from build123d import *

# Parameters (mm, degrees)
REVOLVE1_ANGLE           = 175
REVOLVE1_OTHER_WAY_ANGLE = 175
BOSS_EXTRUDE1_DEPTH      = 1.75
SKETCH5_R                = 1
BOSS_EXTRUDE2_DEPTH      = 3
FILLET1_R                = 1
FILLET1_OF_MIRROR1_R     = 1


with BuildPart() as part:
    # Sketch2 → Revolve1 (revolve)
    with BuildSketch(Plane(origin=(0, 0, 0), x_dir=(0, 0, -1), z_dir=(1, 0, 0))):
        Polygon((1.75, -70), (1.75, -71.8), (1.5, -71.8), (0.5, -73), (-0.5, -73), (-1.5, -71.8), (-1.75, -71.8), (-1.75, -70), align=None)
    revolve(axis=Axis((0, 0, 0), (0, 0, -1)), revolution_arc=REVOLVE1_ANGLE)

    # Sketch2 → Revolve1 other way (revolve)
    with BuildSketch(Plane(origin=(0, 0, 0), x_dir=(0, 0, -1), z_dir=(1, 0, 0))):
        Polygon((1.75, -70), (1.75, -71.8), (1.5, -71.8), (0.5, -73), (-0.5, -73), (-1.5, -71.8), (-1.75, -71.8), (-1.75, -70), align=None)
    revolve(axis=Axis((0, 0, 0), (0, 0, 1)), revolution_arc=REVOLVE1_OTHER_WAY_ANGLE)

    # Sketch3 → Boss-Extrude1 (add, symmetric)
    with BuildSketch(Plane.XY):
        Polygon((-70, 0), (-20, 0), (-20, -3), (-51, -3), (-68.736443607, -13.240140491), (-69.736443607, -11.508089684), (-55, -3), (-70, -3), align=None)
    boss_extrude1 = extrude(amount=BOSS_EXTRUDE1_DEPTH, both=True)

    # Sketch5 → Boss-Extrude2 (add)
    with BuildSketch(Plane(origin=(-20, 0, 0), x_dir=(0, 0, -1), z_dir=(1, 0, 0))):
        with Locations((0, -1.5)):
            Circle(SKETCH5_R)
    boss_extrude2 = extrude(amount=BOSS_EXTRUDE2_DEPTH)

    # Fillet1
    fillet1_edges = [part.edges().sort_by_distance(p)[0] for p in [
        (-69.93568474, -3, 0),
        (-69.107123463, -11.144751529, 0),
        (-70, 0, 0),
        (-55, -3, 0),
        (-51, -3, 0),
    ]]
    fillet(fillet1_edges, radius=FILLET1_R)

    # Mirror1: Boss-Extrude1, Boss-Extrude2 across plane
    add(boss_extrude1.mirror(Plane(origin=(0, 0, 0), x_dir=(0, 0, 1), z_dir=(1, 0, 0))))
    add(boss_extrude2.mirror(Plane(origin=(0, 0, 0), x_dir=(0, 0, 1), z_dir=(1, 0, 0))))

    # Fillet1 of Mirror1
    fillet1_of_mirror1_edges = [part.edges().sort_by_distance(p)[0] for p in [
        (69.93568474, -3, 0),
        (69.107123463, -11.144751529, 0),
        (70, 0, 0),
        (55, -3, 0),
        (51, -3, 0),
    ]]
    fillet(fillet1_of_mirror1_edges, radius=FILLET1_OF_MIRROR1_R)


solid = part.part
Verification items for the finished model (mm, model axes). A direction names the side the tool comes from. Give positions to 0.01 mm unless a question says otherwise; leave off trailing zeros. Use CSV: the item, a comma, the result in double quotes.
1) Release check for a two-part mould opening along X. For faces 1 (the face through (58, -5, -1.75)), 2 (the face through (-45, 0, 0)), 3 (the face through (-3.077, -71.926, 1.34)) record: released by +X, released by -X, zero draft, split by the parting line, or undercut.
Final values:
face 1,"zero draft"
face 2,"undercut"
face 3,"split by the parting line"
2) Go/stop test with flat-tipped pins: pin 1 Ø1.8 at (x, z) = (65, -0.5) entering from -Y; pin 2 Ø0.6 at (y, z) = (-2, 0.5) entering from +X; pin 3 Ø1.5 at (x, z) = (15.5, 0) entering from +Y. Record where each tip stops, or that it passes through.
Final values:
pin 1,"y = -34.93"
pin 2,"x = 72.98"
pin 3,"y = 71.49"
3) Material ranges on line 1 along Y through (x, z) = (55.5, -0.75); line 2 along Y through (x, z) = (26.5, -0.4); line 3 along Y through (x, z) = (-63.5, 0.9), recorded low to high.
Final values:
line 1,"-46.96 to -42.66, -5.6 to 0, 42.66 to 46.96"
line 2,"-68.02 to -64.79, -3 to 0, 64.79 to 68.02"
line 3,"-35.03 to -29.46, -10.22 to -7.91, -3 to 0, 29.46 to 35.03"
4) Access from +Z, -Z, +X, -X, +Y, -Y to the whole of each face (thin tool, end or side, straight path). Record for faces 4 (the face through (69.658, -6.916, -0.024)), 5 (the face through (-3.08, -71.94, -1.33)).
Final values:
face 4,"+Z, -Z"
face 5,"-Z"
5) Cross-section at B-B (x = -42). State how many separate pieces and enclosed holes the cut face has, plus the area to 3 significant figures.
Final values:
separate pieces,"3"
enclosed holes,"0"
area,"32.0 mm²"
